from build123d import *

# Parameters (mm, degrees)
BOSS_EXTRUDE1_DEPTH = 3
BOSS_EXTRUDE2_DEPTH = 33
SHELL2_START        = 2
SHELL2_DEPTH        = 34
SKETCH9_W           = 86.564064606
SKETCH9_H           = 33
SKETCH9_W_2         = 2
CUT_EXTRUDE3_DEPTH  = 3
SKETCH10_W          = 88.564064606
SKETCH10_H          = 33
CUT_EXTRUDE4_DEPTH  = 3
BOSS_EXTRUDE9_DEPTH = 6


# Read off the part's stored shape, not the designer's step: Shell2
with BuildPart() as part:
    # Sketch1 → Boss-Extrude1 (new body)
    with BuildSketch(Plane(origin=(0, 0, 0), x_dir=(1, 0, 0), z_dir=(0, 1, 0))):
        with BuildLine():
            Line((141.421356237, -50), (50, -50))
            Line((50, -50), (50, -141.421356237))
            ThreePointArc((50, -141.421356237), (106.066017178, -106.066017178), (141.421356237, -50))
        make_face()
        with BuildLine():
            Line((50, -50), (30, -50))
            Line((30, -50), (30, -146.969384567))
            ThreePointArc((30, -146.969384567), (40.096074055, -144.541706249), (50, -141.421356237))
            Line((50, -141.421356237), (50, -50))
        make_face()
        with BuildLine():
            Line((50, -30), (50, -50))
            Line((50, -50), (141.421356237, -50))
            ThreePointArc((141.421356237, -50), (144.541706249, -40.096074055), (146.969384567, -30))
            Line((146.969384567, -30), (50, -30))
        make_face()
    extrude(amount=BOSS_EXTRUDE1_DEPTH)

    # Sketch2 → Boss-Extrude2 (add)
    with BuildSketch(Plane(origin=(0, 3, 0), x_dir=(-1, 0, 0), z_dir=(0, 1, 0))):
        with BuildLine():
            Line((-141.421356237, 50), (-50, 50))
            Line((-50, 50), (-50, 141.421356237))
            ThreePointArc((-50, 141.421356237), (-106.066017178, 106.066017178), (-141.421356237, 50))
        make_face()
    extrude(amount=BOSS_EXTRUDE2_DEPTH)

    # Shell2 outline → Shell2 (cut)
    with BuildSketch(Plane(origin=(0, 0, 0), x_dir=(1, 0, 0), z_dir=(0, 1, 0)).offset(SHELL2_START)):
        with BuildLine():
            ThreePointArc((52, -138.564064606), (104.651803616, -104.651803616), (138.564064606, -52))
            Line((138.564064606, -52), (52, -52))
            Line((52, -52), (52, -138.564064606))
        make_face()
    extrude(amount=SHELL2_DEPTH, mode=Mode.SUBTRACT)

    # Sketch9 → Cut-Extrude3 (cut)
    with BuildSketch(Plane.XY.offset(52)):
        with Locations((95.282032303, 19.5)):
            Rectangle(SKETCH9_W, SKETCH9_H)
        with Locations((51, 19.5)):
            Rectangle(SKETCH9_W_2, SKETCH9_H)
    extrude(amount=-CUT_EXTRUDE3_DEPTH, mode=Mode.SUBTRACT)

    # Sketch10 → Cut-Extrude4 (cut)
    with BuildSketch(Plane(origin=(52, 0, 0), x_dir=(0, 0, -1), z_dir=(1, 0, 0))):
        with Locations((-94.282032303, 19.5)):
            Rectangle(SKETCH10_W, SKETCH10_H)
    extrude(amount=-CUT_EXTRUDE4_DEPTH, mode=Mode.SUBTRACT)

    # Sketch11 → Boss-Extrude9 (add)
    with BuildSketch(Plane.XZ):
        with BuildLine():
            ThreePointArc((52, 138.564064606), (104.651803616, 104.651803616), (138.564064606, 52))
            Line((138.564064606, 52), (52, 52))
            Line((52, 52), (52, 138.564064606))
        make_face()
    extrude(amount=-BOSS_EXTRUDE9_DEPTH)


solid = part.part
For this review, take the finished solid that the model builds, in its own axes (mm). A direction names the side the tool comes from. Round coordinates to 2 decimals unless told otherwise and drop trailing zeros. Loops run counter-clockwise (first coordinate to the right, second up) from the corner with the lowest first, then second, coordinate; pieces in that order, holes last. Notation, with made-up numbers: (-27, -35) - (10, -35) arc R8 cw to (10, -25) - close; hole circle Ø5 at (-16.5, 38.25). An arc over 180 degrees is marked (long way). Answer as CSV lines item,"result".
(1) Consider section D-D on x = 46. Give the boundary of the cut face in (y, z).
Checked values:
outline,"(0, 50) - (3, 50) - (3, 142.77) - (0, 142.77) - close"
(2) Consider section B-B on z = 68.5. Give the boundary of the cut face in (x, y).
Checked values:
outline,"(30, 0) - (133.45, 0) - (133.45, 36) - (131.19, 36) - (131.19, 6) - (52, 6) - (52, 3) - (30, 3) - close"
(3) Insertion check: P1, Ø6, axis at y = 4.5, z = 50.5, coming from the +X side; P2, Ø1.5, axis at x = 105.5, y = 5, coming from the -Z side; P3, Ø1.6, axis at x = 51, y = 18, coming from the -Z side. Each pin has a flat end and moves straight along its axis. Give the tip position at first contact, or say it passes through.
Checked values:
P1,"stops at x = 142.15"
P2,"stops at z = 52"
P3,"stops at z = 138.56"
(4) Tool access review of faces 1 (the face through (52, 4, 95)), 2 (the face through (40, 1, 50)), 3 (the face through (50, 19, 140)): name each direction out of +Z, -Z, +X, -X, +Y, -Y from which nothing blocks a thin tool from reaching the whole face with its end or side.
Checked values:
face 1,"-Z, -X, +Y"
face 2,"-Z, -X, +Y, -Y"
face 3,"+Z, -Z, -X, +Y"
(5) Consider section A-A on x = 117. Give the boundary of the cut face in (y, z).
Checked values:
outline,"(0, 30) - (3, 30) - (3, 52) - (6, 52) - (6, 90.64) - (36, 90.64) - (36, 93.87) - (0, 93.87) - close"
(6) Wall thickness on line 1 (Y direction, x = 88.5, z = 39); line 2 (Y direction, x = 116.5, z = 63.5); line 3 (Z direction, x = 119, y = 14): over which ranges is each line inside the solid? List them lowest first.
Checked values:
line 1,"y = 0 to 3"
line 2,"y = 0 to 6"
line 3,"z = 87.99 to 91.32"
(7) Consider section C-C on y = 11. Give the boundary of the cut face in (x, z), then the cut area to 3 significant figures.
Checked values:
outline,"(50, 138.56) - (52, 138.56) arc R148 cw to (138.56, 52) - (138.56, 50) - (141.42, 50) arc R150 ccw to (50, 141.42) - close"
area,"266 mm2"
